Source: CAD feature listing. Evaluate the final solid. Frame: model axes, mm. Face numbers are marked on the shaded views. A direction names the side the tool comes from. Round coordinates to 2 decimals unless told otherwise and drop trailing zeros. Write each loop counter-clockwise with the first axis right and the second up, starting at its lowest first coordinate (ties: lowest second). Pieces come first, ordered by that corner, then holes. Notation, with made-up numbers: M 12,-8 L 62,-8 A38 ccw 62,30 Z; hole C -12,34 d9. An arc over 180 degrees is marked long. Answer in a Markdown table with one row per item.
from build123d import *

# Parameters (mm, degrees)
SKETCH1_R           = 7.5
BOSS_EXTRUDE2_DEPTH = 150
SKETCH1_4_R         = 11.5
SKETCH1_4_R_2       = 7.5
BOSS_EXTRUDE3_DEPTH = 5
SKETCH3_W           = 7
SKETCH3_H           = 7
BOSS_EXTRUDE4_DEPTH = 35
SKETCH7_W           = 5
SKETCH7_H           = 35
CUT_EXTRUDE2_DEPTH  = 10
SKETCH8_R           = 1.5
CUT_EXTRUDE3_DEPTH  = 10


with BuildPart() as part:
    # Sketch1 → Boss-Extrude2 (new body)
    with BuildSketch(Plane.XY):
        Circle(SKETCH1_R)
    extrude(amount=BOSS_EXTRUDE2_DEPTH)

    # Sketch1<4> → Boss-Extrude3 (add)
    with BuildSketch(Plane.XY):
        Circle(SKETCH1_4_R)
        Circle(SKETCH1_4_R_2, mode=Mode.SUBTRACT)
    extrude(amount=BOSS_EXTRUDE3_DEPTH)

    # Sketch3 → Boss-Extrude4 (add)
    with BuildSketch(Plane.XY.offset(150)):
        Rectangle(SKETCH3_W, SKETCH3_H)
    extrude(amount=BOSS_EXTRUDE4_DEPTH)

    # Sketch7 → Cut-Extrude2 (cut)
    with BuildSketch(Plane(origin=(0, 3.5, 0), x_dir=(1, 0, 0), z_dir=(0, 1, 0))):
        with Locations((0, -167.5)):
            Rectangle(SKETCH7_W, SKETCH7_H)
    extrude(amount=-CUT_EXTRUDE2_DEPTH, mode=Mode.SUBTRACT)

    # Sketch8 → Cut-Extrude3 (cut)
    with BuildSketch(Plane(origin=(3.5, 0, 0), x_dir=(0, 0, -1), z_dir=(1, 0, 0))):
        with Locations((-175, 0)):
            Circle(SKETCH8_R)
    extrude(amount=-CUT_EXTRUDE3_DEPTH, mode=Mode.SUBTRACT)


solid = part.part
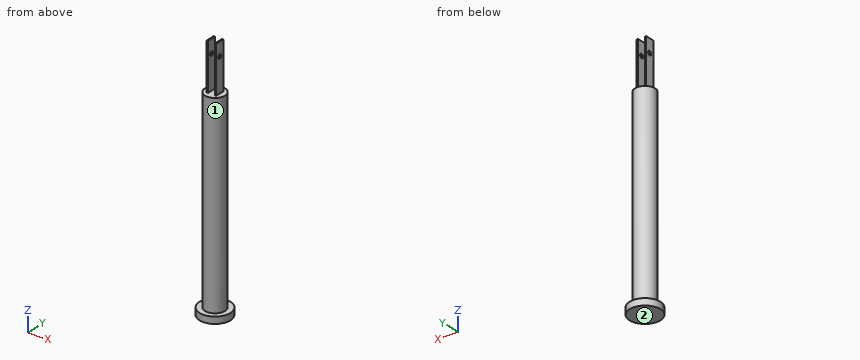
Q1. Section C-C (z = 39). Return loops of the section in (x, y).
Solutions:
| item | result |
|---|---|
| outline | C 0,0 d15 |
Q2. Material intervals for probe 1 along Y at (x, z) = (-2.9, 175); probe 2 along Z at (x, y) = (1.5, -9); probe 3 along Z at (x, y) = (-4, -2), sorted ascending.
Solutions:
| item | result |
|---|---|
| probe 1 | y = -3.5 to -1.5, 1.5 to 3.5 |
| probe 2 | z = 0 to 5 |
| probe 3 | z = 0 to 150 |
Q3. Section B-B (x = 0). Return loops of the section in (y, z), and give its area (3 significant figures).
Solutions:
| item | result |
|---|---|
| outline | M -11.5,0 L 11.5,0 L 11.5,5 L 7.5,5 L 7.5,150 L -7.5,150 L -7.5,5 L -11.5,5 Z |
| area | 2,290 mm2 |
Q4. Section A-A (z = 159.5). Return loops of the section in (x, y).
Solutions:
| item | result |
|---|---|
| outline | M -3.5,-3.5 L -2.5,-3.5 L -2.5,3.5 L -3.5,3.5 Z; M 2.5,-3.5 L 3.5,-3.5 L 3.5,3.5 L 2.5,3.5 Z |
Q5. Access query for the marked faces 1 and 2. Directions: +Z, -Z, +X, -X, +Y, -Y. A direction counts if a zero-diameter tool reaches every point of the face in a straight line with its end or side. Return the directions, or none.
Solutions:
| item | result |
|---|---|
| face 1 | +Z |
| face 2 | -Z, +X, -X, +Y, -Y |
Q6. Section D-D (y = 5.25). Return loops of the section in (x, z), and give its area (3 significant figures).
Solutions:
| item | result |
|---|---|
| outline | M -10.23,0 L 10.23,0 L 10.23,5 L 5.36,5 L 5.36,150 L -5.36,150 L -5.36,5 L -10.23,5 Z |
| area | 1,660 mm2 |
Q7. Contact query for flat-ended pins moving along their axis: pin 1 Ø5 at (x, z) = (2, 39.5) entering from +Y; pin 2 Ø2 at (y, z) = (-7.5, 124) entering from -X; pin 3 Ø1.1 at (x, z) = (3, 167.5) entering from +Y; pin 4 Ø1.5 at (y, z) = (8.5, 38.5) entering from -X. Output: stop coordinate, or through.
Solutions:
| item | result |
|---|---|
| pin 1 | stops at y = 7.5 |
| pin 2 | stops at x = -3.74 |
| pin 3 | stops at y = 3.5 |
| pin 4 | passes through |
